Autodesk Inventor part; units mm, degrees
ref_plane "acrylic_sheet_plane" through (0, 0, 4) normal (0, 0, 1) x (1, 0, 0)
ref_plane "lower test Plane" through (0, 0, 8.5) normal (0, 0, 1) x (1, 0, 0)
ref_plane "YZ Plane" through (0, 0, 0) normal (1, 0, 0) x (0, 1, 0)
sketch "ferrite_layer_outline_sketch" plane through (0, 0, 0) normal (0, 0, 1) x (1, 0, 0)
  line L0 (0, 200) -> (800, 200)
  line L1 (800, 200) -> (800, -200)
  line L2 (800, -200) -> (0, -200)
  line L3 (0, -200) -> (0, 200)
  line L4 (-160, 0) -> (960, 0)
  line L5 (400, 200) -> (400, -200) construction
  line L6 (400, 366.8869) -> (400, -324.3455) construction
  line L7 (400, 200) -> (400, -200)
  point P0 (0, 0)
  point P1 (0, 0)
  point P2 (0, 0)
  point P3 (0, 0)
  point P4 (20, 0)
  dimension "d0" = 800
  dimension "d1" = 400
extrude "Extrusion8" add sketch "ferrite_layer_outline_sketch" along normal blind 4
ref_plane "acrylic_sheet_plane" through (0, 0, 4) normal (0, 0, 1) x (1, 0, 0)
sketch "Sketch4" plane through (0, 0, 4) normal (0, 0, 1) x (1, 0, 0)
  line L0 (14.5, 109) -> (29.5, 109)
  line L1 (29.5, 109) -> (29.5, -109)
  line L2 (29.5, -109) -> (14.5, -109)
  line L3 (14.5, -109) -> (14.5, 109)
  line L4 (-12.6534, 0) -> (47.471, 0)
  line L5 (0, 200) -> (0, -200)
  line L6 (800, 200) -> (0, 200)
  line L7 (0, -200) -> (800, -200)
  point P0 (0, 0)
  point P1 (14.5, 0)
  point P2 (0, 0)
  dimension "d43" = 15
  dimension "d44" = 218
  dimension "d45" = 14.5
extrude "Extrusion9" cut sketch "Sketch4" against normal through all
pattern_linear "Rectangular Pattern 7 fer" count 7 spacing 126 along (1, 0, 0) of "Extrusion9"
pattern_linear "Rectangular Pattern 8 fer" count 8 spacing 108 along (1, 0, 0) of "Extrusion9"
pattern_linear "pattern_test_#_of_ferrites 9 fer" count 9 spacing 94.5 along (1, 0, 0) of "Extrusion9"
pattern_linear "Rectangular Pattern 10 fer" [suppressed]
pattern_linear "Rectangular Pattern 13" count 13 spacing 63 along (1, 0, 0) of "Extrusion9"
sketch "Sketch5" plane through (0, 0, 4) normal (0, 0, 1) x (1, 0, 0)
  line L0 (0, 200) -> (0, -200)
  line L1 (0, 150) -> (800, 150)
  line L2 (800, -200) -> (800, 200)
  line L3 (800, 200) -> (0, 200)
  line L4 (0, -200) -> (800, -200)
  line L5 (0, -150) -> (800, -150)
  point P0 (0, 0)
  dimension "d66" = 50
  dimension "d68" = 50
extrude "Extrusion10" add sketch "Sketch5" along normal blind 4.5 contours L3 L2 L1 L0 | L5 L2 L4 L0
ref_plane "lower test Plane" through (0, 0, 8.5) normal (0, 0, 1) x (1, 0, 0)
sketch "Sketch7" plane through (0, 0, 8.5) normal (0, 0, 1) x (1, 0, 0)
  line L0 (0, 200) -> (0, -200)
  line L1 (0, 175) -> (800, 175)
  line L2 (800, -200) -> (800, 200)
  line L3 (0, -175) -> (800, -175)
  line L4 (800, 200) -> (0, 200)
  line L5 (0, -200) -> (800, -200)
  line L6 (148.5652, 175) -> (148.5652, -175)
  point P0 (0, 0)
  dimension "d77" = 25
  dimension "d78" = 25
extrude "wall extrusion" add sketch "Sketch7" along normal blind 15 contours L4 L2 L1 L0 | L3 L2 L5 L0
extrude "Extrusion14" add sketch "Sketch7" along normal blind 3 contours L1 L6 L3 L0
equation "\"d0\" = track_length"
equation "\"d1\" = track_width"
equation "\"d43\" = ferrite_width"
equation "\"d44\" = ferrite_length"
equation "\"d45\" = gap_distance"
equation "\"d50\" = parameter_5"
equation "\"d62\" = test_parameter_5"
equation "\"track_length\" = 800"
equation "\"track_width\" = 400"
equation "\"gap_distance\" = 14.5"
equation "\"ferrite_length\" = 218"
equation "\"ferrite_width\" = 15"
equation "\"ferrite_height\" = 8"
equation "\"acrylic_sheet_8mm\" = 8"
properties part number "ferrite_layer_dex_0R2"
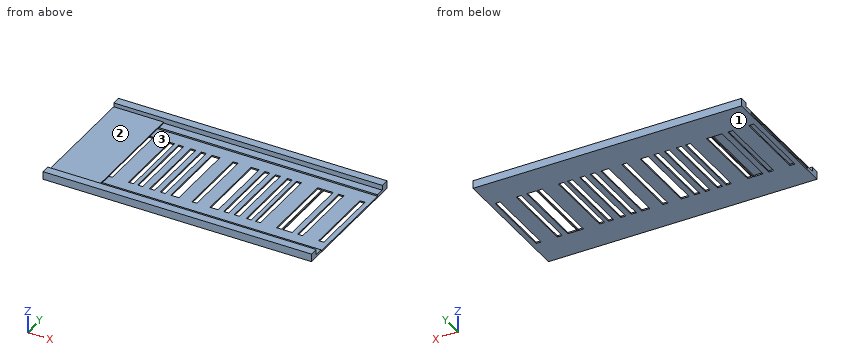
Check sheet for the modelled part. Datum: model origin and axes. Units: mm. Face numbers are marked on the shaded views. Round coordinates to 2 decimals unless told otherwise and drop trailing zeros. Order: outer loops, then holes, each group sorted by start corner. A loop starts at its lowest first (then second) coordinate and runs counter-clockwise, first axis right, second up.
1) Section check C-C (x = 375). Record the boundary of the cut face in (y, z), and give its area (3 significant figures).
2) Scan lines: line 1 (Z direction, x = 96, y = -105.5); line 2 (Y direction, x = 138.5, z = 18.5); line 3 (Y direction, x = 300.5, z = 5). Record each from-to range of solid material in increasing order.
3) Go/stop test with flat-tipped pins: pin 1 Ø1.5 at (y, z) = (-42.5, 10) entering from +X; pin 2 Ø20 at (x, y) = (366, -164) entering from +Z; pin 3 Ø8 at (x, y) = (468, -9) entering from +Z. Record where each tip stops, or that it passes through.
4) Section check A-A (y = 119). Record the boundary of the cut face in (x, z).
5) Mould release check, pull along Z, two halves, no side actions. Record for the marked faces 1, 2 and 3: +Z half, -Z half, draft (parallel to the pull), parting line (faces both ways), or undercut.
6) Section check B-B (z = 16.75). Record the boundary of the cut face in (x, y).
7) Section check D-D (x = 101). Record the boundary of the cut face in (y, z).
Result:
1. outline: (-200, 0) - (200, 0) - (200, 23.5) - (175, 23.5) - (175, 8.5) - (150, 8.5) - (150, 4) - (-150, 4) - (-150, 8.5) - (-175, 8.5) - (-175, 23.5) - (-200, 23.5) - close
1. area: 2,800 mm2
2. line 1: z = 0 to 4, 8.5 to 11.5
2. line 2: y = -200 to -175, 175 to 200
2. line 3: y = -200 to -150, 150 to 200
3. pin 1: stops at x = 148.57
3. pin 2: stops at z = 8.5
3. pin 3: stops at z = 4
4. outline: (0, 0) - (800, 0) - (800, 4) - (0, 4) - close; (0, 8.5) - (148.57, 8.5) - (148.57, 11.5) - (0, 11.5) - close
5. face 1: -Z half
5. face 2: +Z half
5. face 3: undercut
6. outline: (0, -200) - (800, -200) - (800, -175) - (0, -175) - close; (0, 175) - (800, 175) - (800, 200) - (0, 200) - close
7. outline: (-200, 0) - (200, 0) - (200, 23.5) - (175, 23.5) - (175, 11.5) - (-175, 11.5) - (-175, 23.5) - (-200, 23.5) - close; hole (-150, 4) - (150, 4) - (150, 8.5) - (-150, 8.5) - close
